Geometry: see drawing. Coordinates: mm, zero at the bounding-box minimum. A direction names the side the tool comes from. Give positions to 0.01 mm unless a question says otherwise; leave off trailing zeros. Loops run counter-clockwise (first coordinate to the right, second up) from the corner with the lowest first, then second, coordinate; pieces in that order, holes last. Notation, with made-up numbers: (59.5, 34) -> (73.5, 34) arc R25 cw to (73.5, 46) -> close; hole circle Ø2 at (36.5, 60.5). An arc over 180 degrees is marked (long way). Return JSON: item names as keys, results as strings. Group by question number.
(1) Cut plane A-A on x = 22.5. Return loops of the section in (y, z).
(2) Cut plane D-D on y = 15. Return loops of the section in (x, z) (1 decimal).
(3) Ray query, line 1 (Y direction, x = 22.5, z = 16.5); line 2 (Y direction, x = 42, z = 20); line 3 (X direction, y = 15, z = 20). Return the intervals inside material, ascending. Write a range as from..to.
(4) Access query for the marked faces 1 and 2. Directions: +Z, -Z, +X, -X, +Y, -Y. A direction counts if a zero-diameter tool reaches every point of the face in a straight line with its end or side. Return the directions, or none.
(5) Cut plane C-C on x = 10.5. Return loops of the section in (y, z), then the cut area to 3 significant figures.
(6) Cut plane B-B on z = 22.5. Return loops of the section in (x, y) (1 decimal), then the cut area to 3 significant figures.
(7) Pin query (flat end, axial travel): pin 1 (6 mm diameter, centred on x = 28.5, z = 40, fed in from -Y); pin 2 (8 mm diameter, centred on y = 98.5, z = 13.5, fed in from -X); pin 3 (5 mm diameter, centred on y = 37, z = 27, fed in from +X); pin 4 (5.5 mm diameter, centred on x = 22.5, y = 15, fed in from +Z). Return the tip coordinate at first contact, or that it passes through.
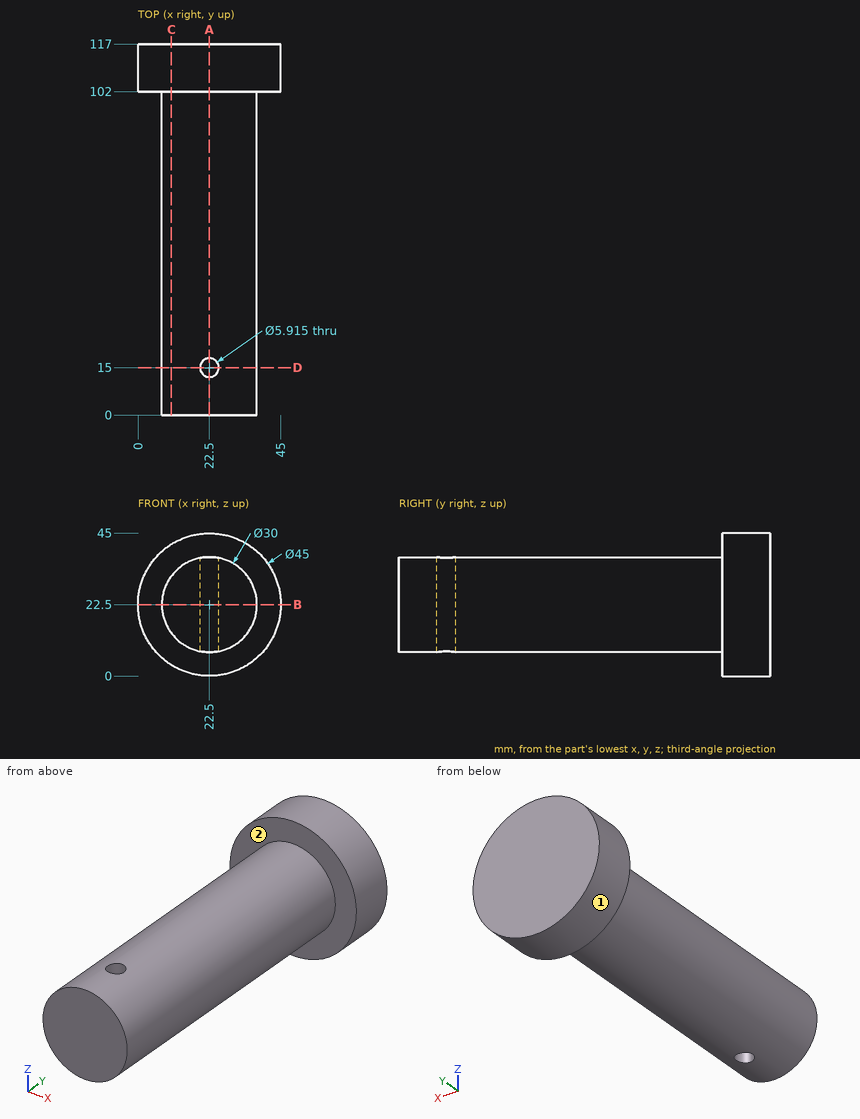
Answers:
{
 "1": {"outline": "(0, 7.5) -> (12.04, 7.5) -> (12.04, 37.5) -> (0, 37.5) -> close; (17.96, 7.5) -> (102, 7.5) -> (102, 0) -> (117, 0) -> (117, 45) -> (102, 45) -> (102, 37.5) -> (17.96, 37.5) -> close"},
 "2": {"outline": "(19.5, 7.8) -> (19.5, 37.2) arc R15 ccw to start; (25.5, 7.8) arc R15 ccw to (25.5, 37.2) -> close"},
 "3": {"line 1": "0..12.04, 17.96..117", "line 2": "102..117", "line 3": "7.71..19.54, 25.46..37.29"},
 "4": {"face 1": "+Y, -Y", "face 2": "-Y"},
 "5": {"outline": "(0, 13.5) -> (102, 13.5) -> (102, 3.47) -> (117, 3.47) -> (117, 41.53) -> (102, 41.53) -> (102, 31.5) -> (0, 31.5) -> close", "area": "2,410 mm²"},
 "6": {"outline": "(0, 102) -> (7.5, 102) -> (7.5, 0) -> (37.5, 0) -> (37.5, 102) -> (45, 102) -> (45, 117) -> (0, 117) -> close; hole circle Ø5.9 at (22.5, 15)", "area": "3,710 mm²"},
 "7": {"pin 1": "y = 102", "pin 2": "x = 1.14", "pin 3": "x = 37.37", "pin 4": "through"}
}
